Verification items for the finished model (mm, model axes). Coordinates: 2 decimals unless noted, no trailing zeros. Loops run counter-clockwise (first coordinate to the right, second up) from the corner with the lowest first, then second, coordinate; pieces in that order, holes last. Notation, with made-up numbers: (-11, 13) -> (33, 13) arc R33 cw to (33, 47) -> close; hole circle Ø9 at (12.25, 49). An arc over 180 degrees is marked (long way). Answer as a JSON object with one key per item and string values. Group by question number.
Q1. Cross-section at B-B on y = 10. Record the boundary of the cut face in (x, z).
Q2. Release check for a two-part mould opening along Y. For faces 1 (the cylindrical face through (-46.792, 10.097, 2.465)), 2 (the cylindrical face through (1.29, 69.99, 2.46)), 3 (the cylindrical face through (65.09, 5.4, 2.54)) record: released by +Y, released by -Y, zero draft, split by the parting line, or undercut.
Q3. Cross-section at D-D on y = 50. Record the boundary of the cut face in (x, z), and give its area (3 significant figures).
Q4. Cross-section at C-C on x = -44.5. Record the boundary of the cut face in (y, z).
Q5. Cross-section at A-A on z = 3.45. Record the boundary of the cut face in (x, y).
Q6. Scan lines: L1, parallel to Y at x = 48, z = 1.55; L2, parallel to Y at x = 1, z = 4.15; L3, parallel to Y at x = -18, z = 0.4. Record each from-to range of solid material in increasing order.
```python
from build123d import *

# Parameters (mm, degrees)
F1_DEPTH = 5
F3_D     = 4.4
F4_R     = 14.224


with BuildPart() as f1:
    # F0 (on Top) → F1 (new body)
    with BuildSketch(Plane.XY):
        with BuildLine():
            Line((-70, 0), (70, 0))
            ThreePointArc((70, 0), (0, 70), (-70, 0))
        make_face()
    extrude(amount=F1_DEPTH)

    # F3 (through all)
    with Locations(Plane.XY.offset(5)):
        with Locations((-34.5178022981, 50), (34.1860465705, 50), (48.9897948557, 10), (-48.9897948557, 10)):
            Hole(F3_D / 2)

    # F4
    f4_edges = [f1.edges().sort_by_distance(p)[0] for p in [
        (70, 0, 2.5),
        (-70, 0, 2.5),
    ]]
    fillet(f4_edges, radius=F4_R)


solid = f1.part
```
Computed values:
{
 "1": {"outline": "(-67.51, 0) -> (-51.19, 0) -> (-51.19, 5) -> (-67.51, 5) -> close; (-46.79, 0) -> (46.79, 0) -> (46.79, 5) -> (-46.79, 5) -> close; (51.19, 0) -> (67.51, 0) -> (67.51, 5) -> (51.19, 5) -> close"},
 "2": {"face 1": "undercut", "face 2": "released by +Y", "face 3": "split by the parting line"},
 "3": {"outline": "(-48.99, 0) -> (-36.72, 0) -> (-36.72, 5) -> (-48.99, 5) -> close; (-32.32, 0) -> (31.99, 0) -> (31.99, 5) -> (-32.32, 5) -> close; (36.39, 0) -> (48.99, 0) -> (48.99, 5) -> (36.39, 5) -> close", "area": "446 mm²"},
 "4": {"outline": "(0, 0) -> (54.03, 0) -> (54.03, 5) -> (0, 5) -> close"},
 "5": {"outline": "(-67.69, 17.85) arc R14.22 ccw to (-53.93, 0) -> (53.93, 0) arc R14.22 ccw to (67.69, 17.85) arc R70 ccw to start; hole circle Ø4.4 at (-48.99, 10); hole circle Ø4.4 at (-34.52, 50); hole circle Ø4.4 at (34.19, 50); hole circle Ø4.4 at (48.99, 10)"},
 "6": {"L1": "y = 0 to 8.04, 11.96 to 50.95", "L2": "y = 0 to 69.99", "L3": "y = 0 to 67.65"}
}
